Solid Edge part; units mm, degrees
sketch "Sketch1" plane through (0, 0, 0) normal (0, 0, 1) x (1, 0, 0)
  line L0 (-25, 15) -> (-25, 0)
  line L1 (-25, 0) -> (-15, 0)
  line L2 (-15, 0) -> (-15, -15)
  line L3 (-15, -15) -> (15, -15)
  line L4 (15, -15) -> (15, 0)
  line L5 (15, 0) -> (25, 0)
  line L6 (25, 0) -> (25, 15)
  line L7 (25, 15) -> (-25, 15)
  dimension "D1" = 25
  dimension "D2" = 15
  dimension "D3" = 15
extrude "Protrusion1" add sketch "Sketch1" along normal mid plane 4
hole "Hole_1" at (-6, -7.5, 2) direction (0, 0, -1) diameter 4 end up to next
hole "Hole1" at (6, -7.5, 2) direction (0, 0, -1) diameter 4 end up to next
chamfer "Chamfer_1" distance 1 angle 45 10 edges at (-25, 7.5, -2) (-20, 0, -2) (-15, -7.5, -2) (0, -15, -2) (15, -7.5, -2) (20, 0, -2) (25, 7.5, -2) (0, 15, -2) (-8, -7.5, -2) (4, -7.5, -2)
hole "Hole_3" at (-15, 7.5, -2) direction (0, 0, 1) diameter 5 end up to next
hole "Hole2" at (15, 7.5, -2) direction (0, 0, 1) diameter 5 end up to next
hole "Hole3" at (0, 7.5, -2) direction (0, 0, 1) diameter 5 end up to next
For this review, take the finished solid that the model builds, in its own axes (mm). A direction names the side the tool comes from. Give positions to 0.01 mm unless a question says otherwise; leave off trailing zeros. Write each loop counter-clockwise with the first axis right and the second up, starting at its lowest first coordinate (ties: lowest second). Pieces come first, ordered by that corner, then holes. Notation, with made-up numbers: M -30,18.5 L 1,18.5 A9 cw 1,34.5 Z; hole C -35,-35 d3. An arc over 180 degrees is marked long. One line per item, written item: value.
1) The part is to be moulded in two halves that separate along X. For faces 4 (the flat face through (-14.5, -6.9, -1.5)), 5 (the cylindrical face through (14.04, 9.81, -0.03)), 6 (the flat face through (-19.4, 0.5, -1.5)), 7 (the cylindrical face through (0.751, 9.885, -0.028)), say which applies: +X half, -X half, draft (parallel to the pull), parting line (faces both ways), or undercut.
Results are:
face 4: -X half
face 5: undercut
face 6: draft
face 7: undercut
2) Take a section at C-C, the plane z = 0.35. Write out the cut boundary in (x, y), then the cut area to 3 significant figures.
Results are:
outline: M -25,0 L -15,0 L -15,-15 L 15,-15 L 15,0 L 25,0 L 25,15 L -25,15 Z; hole C -15,7.5 d5; hole C -6,-7.5 d4; hole C 0,7.5 d5; hole C 6,-7.5 d4; hole C 15,7.5 d5
area: 1,120 mm²
3) Take a section at D-D, the plane y = -11. Write out the cut boundary in (x, z), then the cut area to 3 significant figures.
Results are:
outline: M -15,-1 L -14,-2 L 14,-2 L 15,-1 L 15,2 L -15,2 Z
area: 119 mm²
4) Take a section at A-A, the plane x = 2. Write out the cut boundary in (y, z), then the cut area to 3 significant figures.
Results are:
outline: M -15,-1 L -14,-2 L 6,-2 L 6,2 L -15,2 Z; M 9,-2 L 14,-2 L 15,-1 L 15,2 L 9,2 Z
area: 107 mm²
5) For faces 1 (the flat face through (-0.3, 14.5, -1.5)), 2 (the flat face through (19.4, 0.5, -1.5)), 3 (the flat face through (-20, 0, 0)), list the 3-axis set-ups (+Z, -Z, +X, -X, +Y, -Y) from which the entire face can be reached by the end or side of a thin tool; tool diameter is ignored.
Results are:
face 1: -Z, +X, -X, +Y
face 2: -Z, +X, -Y
face 3: +Z, -Z, -X, -Y
6) Take a section at B-B, the plane y = -7.5. Write out the cut boundary in (x, z).
Results are:
outline: M -15,-1 L -14,-2 L -9,-2 L -8,-1 L -8,2 L -15,2 Z; M -4,-1 L -3,-2 L 3,-2 L 4,-1 L 4,2 L -4,2 Z; M 8,-1 L 9,-2 L 14,-2 L 15,-1 L 15,2 L 8,2 Z
7) For line 1 (X direction, y = -7.5, z = 0.4); line 2 (X direction, y = 7.5, z = -0.75); line 3 (Y direction, x = -6, z = 0.1), list the stretches that pass through material, from the lowest coordinate up. Write a range as from..to.
Results are:
line 1: x = -15..-8, -4..4, 8..15
line 2: x = -25..-17.5, -12.5..-2.5, 2.5..12.5, 17.5..25
line 3: y = -15..-9.5, -5.5..15
8) For P1, Ø4.5, axis at x = -6, y = -7.5, coming from the -Z side; P2, Ø0.9, axis at y = -10.5, z = 0, coming from the +X side; P3, Ø2, axis at y = -7.5, z = 0, coming from the -X side, all flat-tipped, find the tip position at first contact; note any pin that passes through.
Results are:
P1: stops at z = -1.25
P2: stops at x = 15
P3: stops at x = -15
